```python
from build123d import *

# Parameters (mm, degrees)
CUT_EXTRUDE_1_DEPTH      = 31
CUT_EXTRUDE_1_DEPTH_BACK = 31
SKETCH_2_R               = 1.5


with BuildPart() as part:
    # 草图1 → 旋转1 (revolve)
    with BuildSketch(Plane.XY, mode=Mode.PRIVATE) as revolve_1_sk:
        Polygon((-5, 0), (-20, 0), (-20, 3), (-8, 3), (-8, 13), (-5, 13), align=None)
    revolve(revolve_1_sk.sketch.rotate(Axis((0, -573.614855465, 0), (0, 1, 0)), 180), axis=Axis((0, -573.614855465, 0), (0, 1, 0)))

    # 草图2 → 切除-拉伸1 (cut, two sides: drawn at the far end of the back side and taken through both)
    with BuildSketch(Plane(origin=(0, 3, 0), x_dir=(1, 0, 0), z_dir=(0, 1, 0)).offset(-CUT_EXTRUDE_1_DEPTH_BACK)):
        with Locations(Location((0, 15, 0), (0, 0, 180))):
            Circle(SKETCH_2_R)
        with Locations(Location((15, 0, 0), (0, 0, 180))):
            Circle(SKETCH_2_R)
        with Locations(Location((0, -15, 0), (0, 0, 180))):
            Circle(SKETCH_2_R)
        with Locations(Location((-15, 0, 0), (0, 0, 180))):
            Circle(SKETCH_2_R)
    extrude(amount=CUT_EXTRUDE_1_DEPTH + CUT_EXTRUDE_1_DEPTH_BACK, mode=Mode.SUBTRACT)


solid = part.part
```
Here's how the part is built. I have some questions about the finished solid (model axes, mm). A direction names the side the tool comes from. Give positions to 0.01 mm unless a question says otherwise; leave off trailing zeros. Order: outer loops, then holes, each group sorted by start corner. A loop starts at its lowest first (then second) coordinate and runs counter-clockwise, first axis right, second up. Notation, with made-up numbers: (8, 9) -> (53, 9) arc R6 ccw to (53, 13) -> close; hole circle Ø3 at (34, -25.75). An arc over 180 degrees is marked (long way). Use CSV: the item, a comma, the result in double quotes. Start each with the question number.
Item 1: On a 3-axis mill with a long thin cutter (end or side, diameter ignored), from which of +Z, -Z, +X, -X, +Y, -Y can I reach the whole of each face in a straight line? I mean faces 4 (the flat face through (9, 3, 0)), 5 (the cylindrical face through (-5, 6, 0)). Say none if no direction works.
Item 2: Suppose I cut it at D-D (x = 15). List the corners of the cut face in (y, z) for me.
Item 3: Suppose I cut it at B-B (x = 0). List the corners of the cut face in (y, z) for me, and give its area (3 significant figures).
Item 4: If I drill on probe 1 along Z at (x, y) = (0, 2.45); probe 2 along Y at (x, z) = (11.5, 12); probe 3 along Z at (x, y) = (0, 8.5), over which ranges is the centre line in solid material (lowest first)? Write a range as [from, to].
Item 5: I'm going to push flat-ended pins straight in: P1, Ø5, axis at x = 0, z = 15, coming from the +Y side; P2, Ø4, axis at y = 4.5, z = 3, coming from the -X side; P3, Ø6, axis at x = 1, y = 11.5, coming from the +Z side; P4, Ø1.8, axis at x = 0, z = -15, coming from the -Y side. Where does each tip first touch, or does it pass through?
Item 6: Suppose I cut it at C-C (y = 1). List the corners of the cut face in (x, z) for me.
Item 7: Thinking about a two-plate mould opening in X: for faces 1 (the cylindrical face through (-19.98, 1.52, -0.88)), 2 (the flat face through (-4, 0, 4)), 3 (the cylindrical face through (1.11, 1.48, 16.01)), which applies, pulls with the +X half, pulls with the -X half, needs draft (parallel to the pull), parting line crosses it, or undercut?
Item 8: Suppose I cut it at A-A (z = -3.5). List the corners of the cut face in (x, y) for me, and give its area (3 significant figures).
Answer block:
1,face 4,"+Y"
1,face 5,"+Y, -Y"
2,outline,"(0, -13.23) -> (3, -13.23) -> (3, -1.5) -> (0, -1.5) -> close; (0, 1.5) -> (3, 1.5) -> (3, 13.23) -> (0, 13.23) -> close"
3,outline,"(0, -20) -> (3, -20) -> (3, -16.5) -> (0, -16.5) -> close; (0, -13.5) -> (3, -13.5) -> (3, -8) -> (13, -8) -> (13, -5) -> (0, -5) -> close; (0, 5) -> (13, 5) -> (13, 8) -> (3, 8) -> (3, 13.5) -> (0, 13.5) -> close; (0, 16.5) -> (3, 16.5) -> (3, 20) -> (0, 20) -> close"
3,area,"132 mm^2"
4,probe 1,"z = [-20, -16.5], [-13.5, -5], [5, 13.5], [16.5, 20]"
4,probe 2,"y = [0, 3]"
4,probe 3,"z = [-8, -5], [5, 8]"
5,P1,"stops at y = 3"
5,P2,"stops at x = -19.93"
5,P3,"stops at z = 8"
5,P4,"passes through"
6,outline,"circle Ø40 at (0, 0); hole circle Ø3 at (-15, 0); hole circle Ø10 at (0, 0); hole circle Ø3 at (0, -15); hole circle Ø3 at (0, 15); hole circle Ø3 at (15, 0)"
7,face 1,"parting line crosses it"
7,face 2,"needs draft"
7,face 3,"undercut"
8,outline,"(-19.69, 0) -> (-3.57, 0) -> (-3.57, 13) -> (-7.19, 13) -> (-7.19, 3) -> (-19.69, 3) -> close; (3.57, 0) -> (19.69, 0) -> (19.69, 3) -> (7.19, 3) -> (7.19, 13) -> (3.57, 13) -> close"
8,area,"169 mm^2"
